For this review, take the finished solid that the model builds, in its own axes (mm). Face numbers are marked on the shaded views. A direction names the side the tool comes from. Round coordinates to 2 decimals unless told otherwise and drop trailing zeros. Write each loop counter-clockwise with the first axis right and the second up, starting at its lowest first coordinate (ties: lowest second). Pieces come first, ordered by that corner, then holes. Notation, with made-up numbers: (66, -10) -> (102, -10) arc R30 cw to (102, 19) -> close; hole circle Ø2 at (44.5, 5). An arc over 180 degrees is marked (long way). Answer as CSV lines item,"result". Start each with the question number.
Item 1: Take a section at B-B on z = 3.5. Give the boundary of the cut face in (x, y) (3 decimals), then the cut area to 3 significant figures.
Item 2: Wall thickness on probe 1 along Z at (x, y) = (5.5, -4) (3 decimals); probe 2 along X at (y, z) = (-2.75, 5.25) (3 decimals); probe 3 along Z at (x, y) = (0, -0.55) (3 decimals): over which ranges is each line inside the solid? List them lowest first. Write a range as from..to.
Item 3: Mouldability with a two-part tool opening along X and no side actions: class the marked faces 3, 4 and 5 as +X half, -X half, draft (parallel to the pull), parting line (faces both ways), or undercut.
Item 4: Take a section at D-D on z = 8. Give the boundary of the cut face in (x, y) (3 decimals).
Item 5: For pin 1 Ø1.5 at (x, z) = (0.5, -4.5) entering from -Y, flat-tipped, find the tip position at first contact; note if it passes through.
Item 6: Take a section at C-C on y = -5. Count the separate pieces of the cut face and the enclosed holes in it, then the cut area to 3 significant figures.
Item 7: Machinability: for the marked faces 1 and 2, which of the approach directions +Z, -Z, +X, -X, +Y, -Y give a long, thin tool a straight path to every point of the face, cutting with its end or side? Answer none if there is none.
Item 8: Take a section at A-A on x = 0. Give the boundary of the cut face in (y, z) (3 decimals).
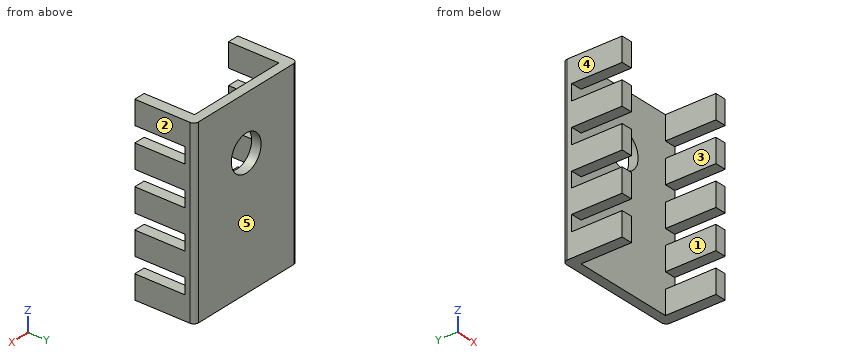
```python
from build123d import *

# Parameters (mm, degrees)
F0_W     = 13.21
F0_H     = 19.05
F1_DEPTH = 1
F2_W     = 1.2
F2_H     = 2.5
F3_DEPTH = 5.35
F4_R     = 0.5
F6_D     = 3.81


with BuildPart() as f1:
    # F0 (on Front) → F1 (new body)
    with BuildSketch(Plane.XZ):
        Rectangle(F0_W, F0_H)
    extrude(amount=F1_DEPTH)

    # F2 (on face) → F3 (join)
    with BuildSketch(Plane.XZ.offset(1)):
        with Locations((6.005, 8.275)):
            Rectangle(F2_W, F2_H)
        with Locations((6.005, 4.125)):
            Rectangle(F2_W, F2_H)
        Polygon((6.605, -1.275), (6.605, 1.225), (5.405, 1.225), (5.405, -1.225), (5.405, -1.275), align=None)
        with Locations((6.005, -4.125)):
            Rectangle(F2_W, F2_H)
        with Locations((6.005, -8.275)):
            Rectangle(F2_W, F2_H)
        with Locations((-6.005, 8.275)):
            Rectangle(F2_W, F2_H)
        with Locations((-6.005, 4.125)):
            Rectangle(F2_W, F2_H)
        with Locations((-6.005, -0.025)):
            Rectangle(F2_W, F2_H)
        with Locations((-6.005, -4.125)):
            Rectangle(F2_W, F2_H)
        with Locations((-6.005, -8.275)):
            Rectangle(F2_W, F2_H)
    extrude(amount=F3_DEPTH)

    # F4
    f4_edges = [f1.edges().sort_by_distance(p)[0] for p in [
        (6.605, 0, 0),
        (-6.605, 0, 0),
    ]]
    fillet(f4_edges, radius=F4_R)

    # F6 (through all)
    with Locations(Plane(origin=(0, 0, 0), x_dir=(-1, 0, 0), z_dir=(0, 1, 0))):
        with Locations((0, 3.805)):
            Hole(F6_D / 2)


solid = f1.part
```
Output values:
1,outline,"(-6.605, -6.35) -> (-5.405, -6.35) -> (-5.405, -1) -> (-1.88, -1) -> (-1.88, 0) -> (-6.105, 0) arc R0.5 ccw to (-6.605, -0.5) -> close; (1.88, -1) -> (5.405, -1) -> (5.405, -6.35) -> (6.605, -6.35) -> (6.605, -0.5) arc R0.5 ccw to (6.105, 0) -> (1.88, 0) -> close"
1,area,"22.2 mm^2"
2,probe 1,"z = -9.525..-7.025, -5.375..-2.875, -1.275..1.225, 2.875..5.375, 7.025..9.525"
2,probe 2,"x = -6.605..-5.405, 5.405..6.605"
2,probe 3,"z = -9.525..1.9, 5.71..9.525"
3,face 3,"undercut"
3,face 4,"-X half"
3,face 5,"draft"
4,outline,"(-6.605, -6.35) -> (-5.405, -6.35) -> (-5.405, -1) -> (5.405, -1) -> (5.405, -6.35) -> (6.605, -6.35) -> (6.605, -0.5) arc R0.5 ccw to (6.105, 0) -> (-6.105, 0) arc R0.5 ccw to (-6.605, -0.5) -> close"
5,pin 1,"stops at y = -1"
6,separate pieces,"10"
6,enclosed holes,"0"
6,area,"30.0 mm^2"
7,face 1,"+Z, -Z, -Y"
7,face 2,"+Z, -Z, +X, +Y, -Y"
8,outline,"(-1, -9.525) -> (0, -9.525) -> (0, 1.9) -> (-1, 1.9) -> close; (-1, 5.71) -> (0, 5.71) -> (0, 9.525) -> (-1, 9.525) -> close"
